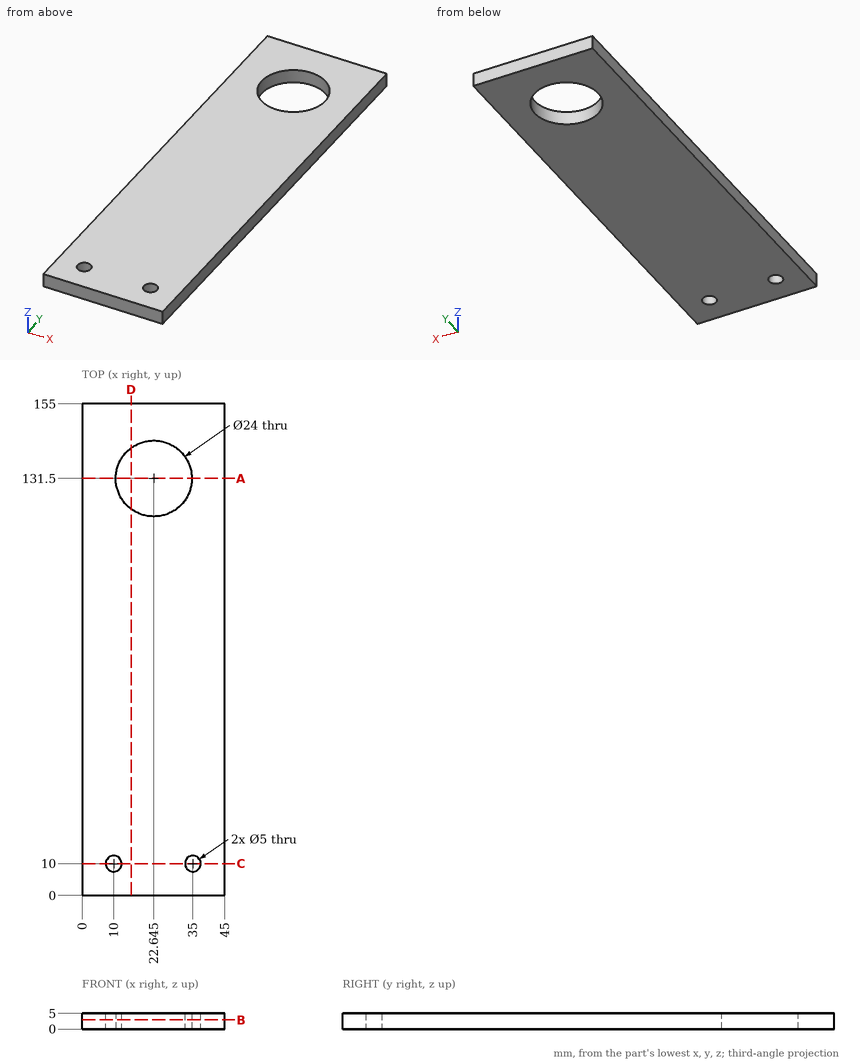
Print and shaded views of the part. All mm, measured from the part's lowest x, y and z. Round coordinates to 2 decimals unless told otherwise and drop trailing zeros. Write each loop counter-clockwise with the first axis right and the second up, starting at its lowest first coordinate (ties: lowest second). Pieces come first, ordered by that corner, then holes.
(1) Slice it at B-B, the plane z = 2.95. Write the cut outline in (x, y) (1 decimal).
(2) Slice it at D-D, the plane x = 15.5. Write the cut outline in (y, z).
(3) Drop flat-ended pins along their axis: P1, Ø4, axis at x = 31, y = 18.5, coming from the -Z side; P2, Ø4, axis at x = 10, y = 10, coming from the -Z side. Give the stop position or say it passes through.
(4) Probe line 1 along X through (y, z) = (10, 2); line 2 along Y through (x, z) = (35, 3.45); line 3 along Y through (x, z) = (15, 3.8). List the from-to ranges inside material, lowest first.
(5) Slice it at A-A, the plane y = 131.5. Write the cut outline in (x, z) (1 decimal), and give its area (3 significant figures).
(6) Slice it at C-C, the plane y = 10. Write the cut outline in (x, z).
From the geometry:
1. outline: (0, 0) - (45, 0) - (45, 155) - (0, 155) - close; hole circle Ø5 at (10, 10); hole circle Ø24 at (22.6, 131.5); hole circle Ø5 at (35, 10)
2. outline: (0, 0) - (121.86, 0) - (121.86, 5) - (0, 5) - close; (141.14, 0) - (155, 0) - (155, 5) - (141.14, 5) - close
3. P1: stops at z = 0
3. P2: passes through
4. line 1: x = 0 to 7.5, 12.5 to 32.5, 37.5 to 45
4. line 2: y = 0 to 7.5, 12.5 to 155
4. line 3: y = 0 to 122.25, 140.75 to 155
5. outline: (0, 0) - (10.6, 0) - (10.6, 5) - (0, 5) - close; (34.6, 0) - (45, 0) - (45, 5) - (34.6, 5) - close
5. area: 105 mm2
6. outline: (0, 0) - (7.5, 0) - (7.5, 5) - (0, 5) - close; (12.5, 0) - (32.5, 0) - (32.5, 5) - (12.5, 5) - close; (37.5, 0) - (45, 0) - (45, 5) - (37.5, 5) - close
